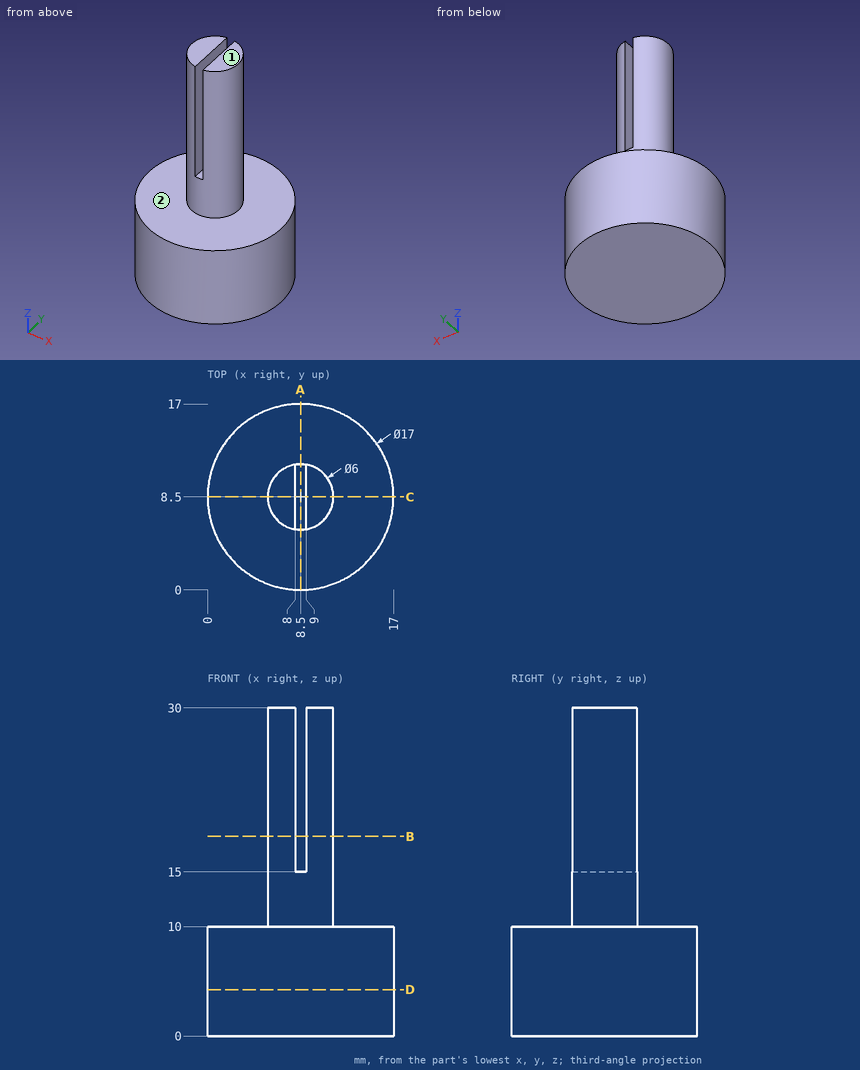
Design review of the part shown in the three views and the two pictorial views. Dimensions are in mm from the part's minimum x, y and z. A direction names the side the tool comes from. Round coordinates to 2 decimals unless told otherwise and drop trailing zeros. Order: outer loops, then holes, each group sorted by start corner. A loop starts at its lowest first (then second) coordinate and runs counter-clockwise, first axis right, second up. Notation, with made-up numbers: M 61,-1.75 L 81,-1.75 A22 ccw 81,23.25 Z; hole C 4,-7 d2. An arc over 180 degrees is marked long. Put each result on its own line as item: value.
Q1. Consider section A-A (x = 8.5). State the section outline as (y, z) points.
Reported:
outline: M 0,0 L 17,0 L 17,10 L 11.5,10 L 11.5,15 L 5.5,15 L 5.5,10 L 0,10 Z
Q2. Insertion check: pin 1 Ø1.5 at (y, z) = (7, 22) entering from -X; pin 2 Ø8 at (x, y) = (3, 11.5) entering from -Z; pin 3 Ø1.5 at (y, z) = (11, 12) entering from -X; pin 4 Ø3 at (y, z) = (9.5, 24.5) entering from +X. Each pin has a flat end and moves straight along its axis. Give the tip position at first contact, or say it passes through.
Reported:
pin 1: x = 5.6
pin 2: z = 0
pin 3: x = 6.06
pin 4: x = 11.5
Q3. Consider section B-B (z = 18.25). State the section outline as (x, y) points.
Reported:
outline: M 8,5.54 L 8,11.46 A3 ccw Z; M 9,5.54 A3 ccw 9,11.46 Z
Q4. Consider section D-D (z = 4.25). State the section outline as (x, y) points.
Reported:
outline: C 8.5,8.5 d17
Q5. Machinability: for the marked faces 1 and 2, which of the approach directions +Z, -Z, +X, -X, +Y, -Y give a long, thin tool a straight path to every point of the face, cutting with its end or side? Answer none if there is none.
Reported:
face 1: +Z, +X, -X, +Y, -Y
face 2: +Z
Q6. To check wall thickness, follow line 1 (Z direction, x = 3.25, y = 11.75); line 2 (Y direction, x = 9.75, z = 21); line 3 (X direction, y = 8.25, z = 24). State the ranges of each line that lie inside material, in increasing order.
Reported:
line 1: 0 to 10
line 2: 5.77 to 11.23
line 3: 5.51 to 8, 9 to 11.49
Q7. Consider section C-C (y = 8.5). State the section outline as (x, z) points, and give its area (3 significant figures).
Reported:
outline: M 0,0 L 17,0 L 17,10 L 11.5,10 L 11.5,30 L 9,30 L 9,15 L 8,15 L 8,30 L 5.5,30 L 5.5,10 L 0,10 Z
area: 275 mm²
